from build123d import *

# Parameters (mm, degrees)
F1_DEPTH = 57.15


with BuildPart() as f1:
    # F0 (on Top) → F1 (new body)
    with BuildSketch(Plane.XY):
        with BuildLine():
            ThreePointArc((0, 1.5875), (0.464968, 0.464968), (1.5875, 0))
            Line((1.5875, 0), (34.925, 0))
            Line((34.925, 0), (33.535938, 3.175))
            Line((33.535938, 3.175), (13.11615, 49.8488))
            ThreePointArc((13.11615, 49.8488), (12.530666, 50.541086), (11.66175, 50.8))
            Line((11.66175, 50.8), (1.5875, 50.8))
            ThreePointArc((1.5875, 50.8), (0.464968, 50.335032), (0, 49.2125))
            Line((0, 49.2125), (0, 1.5875))
        make_face()
        with BuildLine():
            ThreePointArc((4.7625, 3.175), (3.639968, 3.639968), (3.175, 4.7625))
            Line((3.175, 4.7625), (3.175, 46.0375))
            ThreePointArc((3.175, 46.0375), (3.639968, 47.160032), (4.7625, 47.625))
            Line((4.7625, 47.625), (9.585251, 47.625))
            ThreePointArc((9.585251, 47.625), (10.454167, 47.366086), (11.039651, 46.6738))
            Line((11.039651, 46.6738), (29.097463, 5.3988))
            ThreePointArc((29.097463, 5.3988), (28.971649, 3.893584), (27.643063, 3.175))
            Line((27.643063, 3.175), (4.7625, 3.175))
        make_face(mode=Mode.SUBTRACT)
        with BuildLine():
            Line((33.535938, 3.175), (34.925, 0))
            Line((34.925, 0), (52.3875, 0))
            ThreePointArc((52.3875, 0), (53.510032, 0.464968), (53.975, 1.5875))
            Line((53.975, 1.5875), (53.975, 9.525))
            ThreePointArc((53.975, 9.525), (53.510032, 10.647532), (52.3875, 11.1125))
            ThreePointArc((52.3875, 11.1125), (51.264968, 10.647532), (50.8, 9.525))
            Line((50.8, 9.525), (50.8, 3.175))
            Line((50.8, 3.175), (33.535938, 3.175))
        make_face()
    extrude(amount=F1_DEPTH)


solid = f1.part
For this review, take the finished solid that the model builds, in its own axes (mm). A direction names the side the tool comes from. Round coordinates to 2 decimals unless told otherwise and drop trailing zeros. Order: outer loops, then holes, each group sorted by start corner. A loop starts at its lowest first (then second) coordinate and runs counter-clockwise, first axis right, second up. Notation, with made-up numbers: M 74.25,34 L 105.25,34 A14 ccw 105.25,57 Z; hole C -25.5,78.5 d2. An arc over 180 degrees is marked long. Use a Markdown table: item, result. Add a question column.
Item 1: To check wall thickness, follow line 1 along X through (y, z) = (42.5, 22.5) (3 decimals); line 2 along X through (y, z) = (24, 7) (3 decimals); line 3 along Y through (x, z) = (16, 38) (3 decimals). State the ranges of each line that lie inside material, in increasing order.
Item 2: Insertion check: pin 1 (5 mm diameter, centred on x = 43.5, z = 28, fed in from +Y) (3 decimals); pin 2 (2 mm diameter, centred on y = 33, z = 19, fed in from +X) (3 decimals); pin 3 (12.5 mm diameter, centred on y = 24, z = 14.5, fed in from +X). Each pin has a flat end and moves straight along its axis. Give the tip position at first contact, or say it passes through.
Item 3: Mouldability with a two-part tool opening along X and no side actions: class faces 1 (the flat face through (3.175, 25, 28)), 2 (the flat face through (27, 0, 28)), 3 (the cylindrical face through (0.45, 0.48, 28.17)), 4 (the flat face through (42, 3.175, 28)) as released by +X, released by -X, zero draft, split by the parting line, or undercut.
Item 4: Add section D-D, the plane y = 23.5. Give the boundary of the cut face in (x, z) (3 decimals), then the cut area to 3 significant figures.
Item 5: Add section A-A, the plane x = 6. Give the boundary of the cut face in (y, z) (3 decimals).
Item 6: Add section B-B, the plane y = 6.5. Give the boundary of the cut face in (x, z) (3 decimals), then the cut area to 3 significant figures.
Item 7: Tool access review of faces 5 (the cylindrical face through (10.4, 47.4, 28.2)), 6 (the cylindrical face through (0.48, 50.35, 28.17)), 7 (the flat face through (50.8, 6, 28)): name each direction out of +Z, -Z, +X, -X, +Y, -Y from which nothing blocks a thin tool from reaching the whole face with its end or side.
Item 8: Add section C-C, the plane z = 40.5. Give the boundary of the cut face in (x, y) (1 decimal), then the cut area to 3 significant figures.
Geometry results:
| question | item | result |
|---|---|---|
| 1 | line 1 | x = 0 to 3.175, 12.866 to 16.331 |
| 1 | line 2 | x = 0 to 3.175, 20.959 to 24.425 |
| 1 | line 3 | y = 0 to 3.175, 35.336 to 43.257 |
| 2 | pin 1 | stops at y = 3.175 |
| 2 | pin 2 | stops at x = 20.925 |
| 2 | pin 3 | stops at x = 27.16 |
| 3 | face 1 | undercut |
| 3 | face 2 | zero draft |
| 3 | face 3 | released by -X |
| 3 | face 4 | undercut |
| 4 | outline | M 0,0 L 3.175,0 L 3.175,57.15 L 0,57.15 Z; M 21.178,0 L 24.644,0 L 24.644,57.15 L 21.178,57.15 Z |
| 4 | area | 380 mm² |
| 5 | outline | M 0,0 L 3.175,0 L 3.175,57.15 L 0,57.15 Z; M 47.625,0 L 50.8,0 L 50.8,57.15 L 47.625,57.15 Z |
| 6 | outline | M 0,0 L 3.175,0 L 3.175,57.15 L 0,57.15 Z; M 28.616,0 L 32.081,0 L 32.081,57.15 L 28.616,57.15 Z; M 50.8,0 L 53.975,0 L 53.975,57.15 L 50.8,57.15 Z |
| 6 | area | 561 mm² |
| 7 | face 5 | +Z, -Z |
| 7 | face 6 | +Z, -Z, -X, +Y |
| 7 | face 7 | +Z, -Z, +Y |
| 8 | outline | M 0,1.6 A1.6 ccw 1.6,0 L 52.4,0 A1.6 ccw 54,1.6 L 54,9.5 A1.6 ccw 50.8,9.5 L 50.8,3.2 L 33.5,3.2 L 13.1,49.8 A1.6 ccw 11.7,50.8 L 1.6,50.8 A1.6 ccw 0,49.2 Z; hole M 3.2,4.8 A1.6 ccw 4.8,3.2 L 27.6,3.2 A1.6 ccw 29.1,5.4 L 11,46.7 A1.6 ccw 9.6,47.6 L 4.8,47.6 A1.6 ccw 3.2,46 Z |
| 8 | area | 534 mm² |
